For this review, take the finished solid that the model builds, in its own axes (mm). A direction names the side the tool comes from. Give positions to 0.01 mm unless a question says otherwise; leave off trailing zeros. Loops run counter-clockwise (first coordinate to the right, second up) from the corner with the lowest first, then second, coordinate; pieces in that order, holes last.
```python
from build123d import *

# Parameters (mm, degrees)
BOSS_EXTRUDE2_DEPTH = 15
BOSS_EXTRUDE3_DEPTH = 5
BOSS_EXTRUDE4_DEPTH = 5
BOSS_EXTRUDE5_DEPTH = 10
SKETCH10_W          = 10
SKETCH10_H          = 3
BOSS_EXTRUDE6_DEPTH = 5.3
FILLET1_R           = 2
FILLET2_R           = 2


with BuildPart() as part:
    # Sketch2 → Boss-Extrude2 (new, symmetric)
    with BuildSketch(Plane(origin=(0, 0, 0), x_dir=(0, 0, -1), z_dir=(1, 0, 0))):
        Polygon((0, 0), (0, -40), (5, -40), (5, -7), (40, -7), (40, 0), align=None)
    extrude(amount=BOSS_EXTRUDE2_DEPTH, both=True)

    # Sketch3 → Boss-Extrude3 (add, symmetric)
    with BuildSketch(Plane(origin=(0, 0, 0), x_dir=(0, 0, -1), z_dir=(1, 0, 0))):
        Polygon((0, -116), (-15, -116), (-15, 32.97157442), (0, 55.00157442), align=None)
    extrude(amount=BOSS_EXTRUDE3_DEPTH, both=True)

    # Sketch4 → Boss-Extrude4 (add)
    with BuildSketch(Plane.ZY.offset(5)):
        Polygon((0, 60), (20.3, 60), (20.3, -116), (0, -116), (0, 0), (-5, 0), (-5, 60), align=None)
    boss_extrude4 = extrude(amount=BOSS_EXTRUDE4_DEPTH)

    # Mirror1: Boss-Extrude4 across plane
    add(boss_extrude4.mirror(Plane(origin=(0, 0, 0), x_dir=(0, 0, 1), z_dir=(1, 0, 0))))

    # Sketch8 → Boss-Extrude5 (add)
    with BuildSketch(Plane.ZY.offset(-5)):
        Polygon((0, 0), (0, 55), (20.3, 55), (20.3, 58.7), (-9.7, 58.7), (-9.7, 0), align=None)
    extrude(amount=BOSS_EXTRUDE5_DEPTH)

    # Sketch10 → Boss-Extrude6 (add)
    with BuildSketch(Plane.XY.offset(15)):
        with Locations((0, -114.5)):
            Rectangle(SKETCH10_W, SKETCH10_H)
    extrude(amount=BOSS_EXTRUDE6_DEPTH)

    # Fillet1
    # the kernel refuses this fillet: 2 mm, written as the material it takes off along each edge
    with BuildSketch(Plane(origin=(5, 58.7, 20.3), x_dir=(0, -1, 0), z_dir=(-1, 0, 0))) as fillet1_piece_1:
        with BuildLine():
            CenterArc((FILLET1_R, -FILLET1_R), FILLET1_R, 90, 90)
            Line((0, -FILLET1_R), (0, 0))
            Line((0, 0), (FILLET1_R, 0))
        make_face()
    extrude(amount=10, mode=Mode.SUBTRACT)
    with BuildSketch(Plane(origin=(10, 58.7, -9.7), x_dir=(0, 0, 1), z_dir=(-1, 0, 0))) as fillet1_piece_2:
        with BuildLine():
            CenterArc((FILLET1_R, -FILLET1_R), FILLET1_R, 90, 90)
            Line((0, -FILLET1_R), (0, 0))
            Line((0, 0), (FILLET1_R, 0))
        make_face()
    extrude(amount=20, mode=Mode.SUBTRACT)
    with BuildSketch(Plane(origin=(-5, 60, -5), x_dir=(0, -1, 0), z_dir=(-1, 0, 0)), Plane(origin=(5, 60, -5), x_dir=(0, 0, 1), z_dir=(1, 0, 0))) as fillet1_piece_3:
        with BuildLine():
            CenterArc((FILLET1_R, FILLET1_R), FILLET1_R, 180, 90)
            Line((0, FILLET1_R), (0, 0))
            Line((0, 0), (FILLET1_R, 0))
        make_face()
    extrude(amount=10, mode=Mode.SUBTRACT)

    # Fillet2
    fillet2_edges = [part.edges().sort_by_distance(p)[0] for p in [
        (12.5, 0, 0),
        (-12.5, 0, 0),
    ]]
    fillet(fillet2_edges, radius=FILLET2_R)


solid = part.part
```
Item 1: Take a section at B-B on x = -1.5. Give the boundary of the cut face in (y, z).
Answer:
outline: (-116, 0) - (-40, 0) - (-40, -5) - (-7, -5) - (-7, -40) - (0, -40) - (0, -9.7) - (56.7, -9.7) arc R2 ccw to (58.7, -7.7) - (58.7, 18.3) arc R2 ccw to (56.7, 20.3) - (55, 20.3) - (55, 0) - (32.97, 15) - (-113, 15) - (-113, 20.3) - (-116, 20.3) - close
Item 2: For L1, parallel to X at y = 39.5, z = 14; L2, parallel to Z at x = -2.25, y = -79.5; L3, parallel to Y at x = -5.25, z = -36, list the stretches that pass through material, from the lowest coordinate up.
Answer:
L1: x = -10 to -5, 5 to 10
L2: z = 0 to 15
L3: y = -7 to 0
Item 3: The part is to be moulded in two halves that separate along Y. For faces 1 (the flat face through (-15, -6.6, -15.5)), 2 (the flat face through (0, -7, -22)), 3 (the flat face through (0, -113, 18)), say which applies: released by +Y, released by -Y, zero draft, split by the parting line, or undercut.
Answer:
face 1: zero draft
face 2: released by -Y
face 3: undercut
Item 4: Tool access review of faces 4 (the flat face through (5, -16, 17)), 5 (the flat face through (0, 58.7, 5)), 6 (the flat face through (5, 29, -7)), 7 (the flat face through (-7, 29, -5)): name each direction out of +Z, -Z, +X, -X, +Y, -Y from which nothing blocks a thin tool from reaching the whole face with its end or side.
Answer:
face 4: +Z
face 5: +Z, -Z, +Y
face 6: -Z, +X, +Y
face 7: -Z, -X, +Y
Item 5: Take a section at A-A on y = -53. Give the boundary of the cut face in (x, z), and give its area (3 significant figures).
Answer:
outline: (-10, 0) - (10, 0) - (10, 20.3) - (5, 20.3) - (5, 15) - (-5, 15) - (-5, 20.3) - (-10, 20.3) - close
area: 353 mm2
Item 6: Take a section at C-C on y = -30. Give the boundary of the cut face in (x, z).
Answer:
outline: (-15, -5) - (15, -5) - (15, 0) - (10, 0) - (10, 20.3) - (5, 20.3) - (5, 15) - (-5, 15) - (-5, 20.3) - (-10, 20.3) - (-10, 0) - (-15, 0) - close
Item 7: Take a section at D-D on z = -26.5. Give the boundary of the cut face in (x, y), and give its area (3 significant figures).
Answer:
outline: (-15, -7) - (15, -7) - (15, 0) - (-15, 0) - close
area: 210 mm2
Item 8: Clearance check with flat-ended pins moving along their axes: pin 1 Ø1 at (y, z) = (59, 9.5) entering from +X; pin 2 Ø16 at (x, y) = (3, -62) entering from -Z; pin 3 Ø8 at (x, y) = (0, 26.5) entering from -Z; pin 4 Ø4 at (x, z) = (7, -1.5) entering from -Y. State where each tip first meets the part, or that it passes through.
Answer:
pin 1: stops at x = 10
pin 2: stops at z = 0
pin 3: stops at z = -9.7
pin 4: stops at y = -116
